Could you check a few things on this model? Use its own coordinates, in mm. Face numbers are marked on the shaded views. Coordinates: 2 decimals unless noted, no trailing zeros. Order: outer loops, then holes, each group sorted by start corner. A loop starts at its lowest first (then second) coordinate and runs counter-clockwise, first axis right, second up. Notation, with made-up numbers: M 27,-34 L 77,-34 A27 ccw 77,-6 Z; hole C 13,4 d7. An arc over 180 degrees is marked long. Put each result on its own line as item: value. Start each with the question number.
```python
from build123d import *

# Parameters (mm, degrees)
F0_R     = 6.25
F1_DEPTH = 1
F2_R     = 6.25
F2_R_2   = 5.75
F3_DEPTH = 0.75
F4_R     = 4
F5_DEPTH = 14.5
F6_R     = 3.5
F7_DEPTH = 25
F8_SIZE  = 0.3


with BuildPart() as f1:
    # F0 (on Top) → F1 (new body)
    with BuildSketch(Plane.XY):
        Circle(F0_R)
    extrude(amount=F1_DEPTH)

    # F2 (on face) → F3 (join)
    with BuildSketch(Plane(origin=(0, 0, 0), x_dir=(1, 0, 0), z_dir=(0, 0, -1))):
        Circle(F2_R)
        Circle(F2_R_2, mode=Mode.SUBTRACT)
    extrude(amount=F3_DEPTH)

    # F4 (on face) → F5 (join)
    with BuildSketch(Plane.XY.offset(1)):
        Circle(F4_R)
    extrude(amount=F5_DEPTH)

    # F6 (on face) → F7 (cut)
    with BuildSketch(Plane.XY.offset(15.5)):
        Circle(F6_R)
    extrude(amount=-F7_DEPTH, mode=Mode.SUBTRACT)

    # F8
    f8_edges = [f1.edges().sort_by_distance(p)[0] for p in [
        (-5.75, 0, -0.75),
    ]]
    chamfer(f8_edges, length=F8_SIZE)


solid = f1.part
```
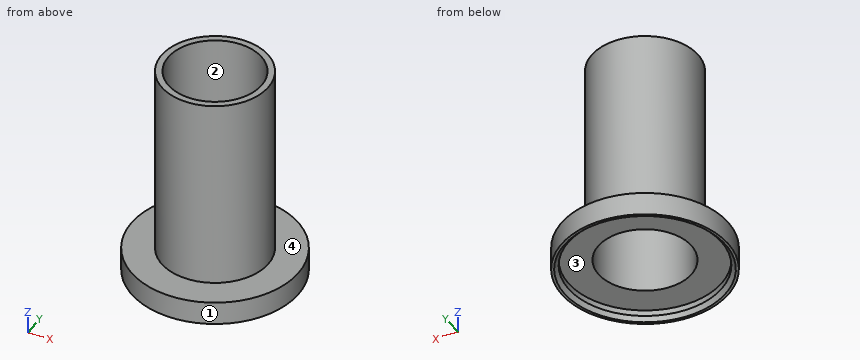
Item 1: If we section it at A-A on x = 0: Write out the boundary of the cut face in (y, z).
Item 2: For pin 1 Ø3.5 at (x, y) = (-2.5, -1.5) entering from -Z; pin 2 Ø5 at (x, z) = (-4, 13.5) entering from +Y; pin 3 Ø1 at (y, z) = (-1, 11.5) entering from +X, each with a flat end and sliding along its axis, tell me the tip position at first contact or that it passes through.
Item 3: If we section it at C-C on z = 14.75: Write out the boundary of the cut face in (x, y), then the cut area to 3 significant figures.
Item 4: I need wall thicknesses on probe 1 along Y at (x, z) = (0, 6.75); probe 2 along X at (y, z) = (0, -0.05). Which ranges of each line are inside material? Lowest first, please.
Item 5: If we mould it in two halves opening along Y, with no side actions, what happens to the marked faces 1, 2, 3 and 4? For each: released by +Y, released by -Y, zero draft, split by the parting line, or undercut.
Geometry check:
1. outline: M -6.25,-0.75 L -6.05,-0.75 L -5.75,-0.45 L -5.75,0 L -3.5,0 L -3.5,15.5 L -4,15.5 L -4,1 L -6.25,1 Z; M 3.5,0 L 5.75,0 L 5.75,-0.45 L 6.05,-0.75 L 6.25,-0.75 L 6.25,1 L 4,1 L 4,15.5 L 3.5,15.5 Z
2. pin 1: stops at z = 0
2. pin 2: stops at y = 3.71
2. pin 3: stops at x = 3.97
3. outline: C 0,0 d8; hole C 0,0 d7
3. area: 11.8 mm²
4. probe 1: y = -4 to -3.5, 3.5 to 4
4. probe 2: x = -6.25 to -5.75, 5.75 to 6.25
5. face 1: split by the parting line
5. face 2: undercut
5. face 3: undercut
5. face 4: zero draft
